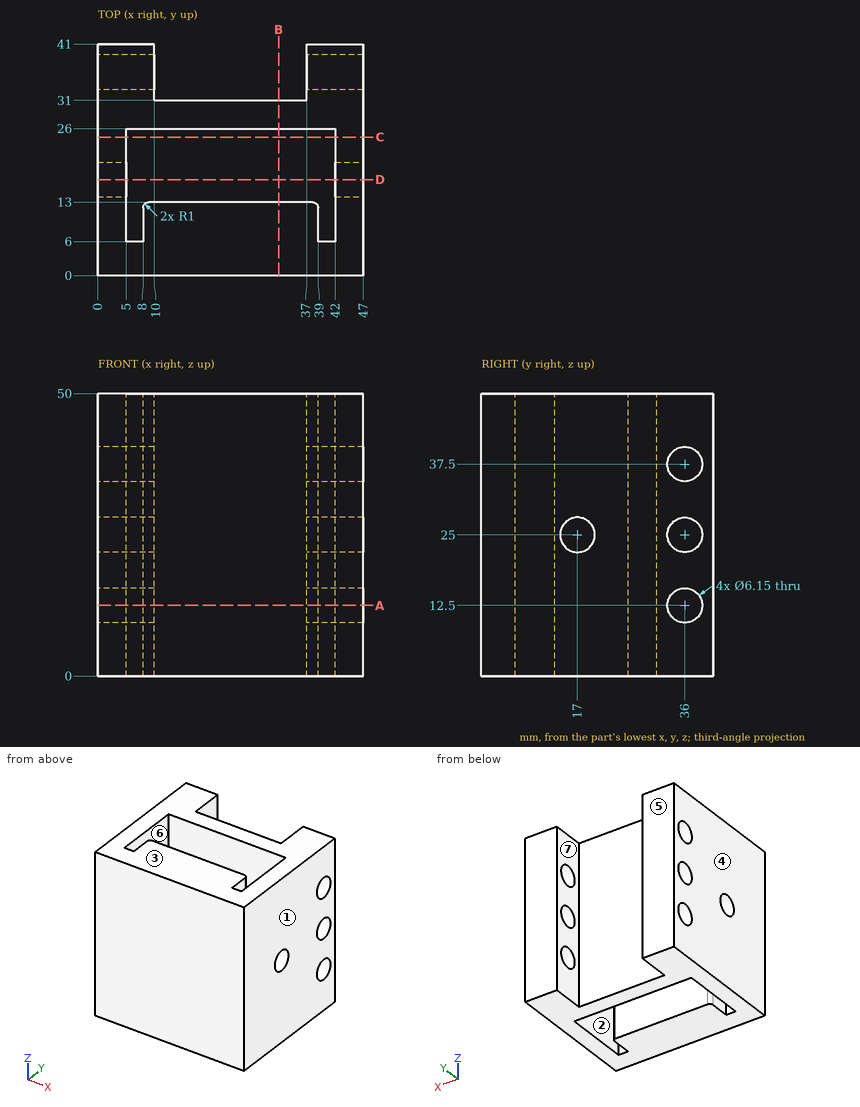
Source: three-view drawing plus pictorial views. Frame: mm from the lowest corner of the part. A direction names the side the tool comes from. Round coordinates to 2 decimals unless told otherwise and drop trailing zeros. Write each loop counter-clockwise with the first axis right and the second up, starting at its lowest first coordinate (ties: lowest second). Pieces come first, ordered by that corner, then holes. Notation, with made-up numbers: M 80.5,53.5 L 104.5,53.5 A19 cw 104.5,62.5 Z; hole C 33.25,71.5 d6. An arc over 180 degrees is marked long. One line per item, written item: value. Start each with the question number.
Item 1: Section query C-C (y = 24.5). Return the cut outline in (x, z), plus the area to 3 significant figures.
Item 2: Section query B-B (x = 32). Return the cut outline in (y, z), plus the area to 3 significant figures.
Item 3: Ray query, L1, parallel to Z at x = 4.75, y = 36 (3 decimals); L2, parallel to Y at x = 3.85, z = 25 (3 decimals); L3, parallel to X at y = 10, z = 36.5. Return the intervals inside material, ascending. Write a range as from..to.
Item 4: Set-up query: the marked faces 5, 6 and 7. Return all of +Z, -Z, +X, -X, +Y, -Y with unobstructed straight access to the full face (end or side cutting, diameter ignored); none if empty.
Item 5: Mould query, pull axis X, two halves, no side actions, for the marked faces 1, 2, 3 and 4. Classes: pulls with the +X half, pulls with the -X half, needs draft (parallel to the pull), parting line crosses it, or undercut.
Item 6: Section query A-A (z = 12.5). Return the cut outline in (x, y) (3 decimals), plus the area to 3 significant figures.
Item 7: Pin query (flat end, axial travel): pin 1 (8 mm diameter, centred on x = 20, z = 30, fed in from +Y). Return the tip coordinate at first contact, or that it passes through.
Item 8: Section query D-D (y = 17). Return the cut outline in (x, z) (3 decimals).
Result set:
1. outline: M 0,0 L 5,0 L 5,50 L 0,50 Z; M 42,0 L 47,0 L 47,50 L 42,50 Z
1. area: 500 mm²
2. outline: M 0,0 L 13,0 L 13,50 L 0,50 Z; M 26,0 L 31,0 L 31,50 L 26,50 Z
2. area: 900 mm²
3. L1: z = 0..9.425, 15.575..21.925, 28.075..34.425, 40.575..50
3. L2: y = 0..13.925, 20.075..32.925, 39.075..41
3. L3: x = 0..5, 8..39, 42..47
4. face 5: +Z, -Z, +X, -X, +Y
4. face 6: +Z, -Z
4. face 7: +Z, -Z, +Y
5. face 1: pulls with the +X half
5. face 2: undercut
5. face 3: needs draft
5. face 4: pulls with the -X half
6. outline: M 0,0 L 47,0 L 47,32.925 L 37,32.925 L 37,31 L 10,31 L 10,32.925 L 0,32.925 Z; M 0,39.075 L 10,39.075 L 10,41 L 0,41 Z; M 37,39.075 L 47,39.075 L 47,41 L 37,41 Z; hole M 5,6 L 8,6 L 8,12 A1 cw 9,13 L 38,13 A1 cw 39,12 L 39,6 L 42,6 L 42,26 L 5,26 Z
6. area: 1,010 mm²
7. pin 1: stops at y = 31
8. outline: M 0,0 L 5,0 L 5,21.925 L 0,21.925 Z; M 0,28.075 L 5,28.075 L 5,50 L 0,50 Z; M 42,0 L 47,0 L 47,21.925 L 42,21.925 Z; M 42,28.075 L 47,28.075 L 47,50 L 42,50 Z
